from build123d import *

# Parameters (mm, degrees)
F2_R     = 32
F2_R_2   = 12
F3_DEPTH = 5
F4_R     = 5
F5_DEPTH = 5


with BuildPart() as f1:
    # F0 (on Front) → F1 (revolve)
    with BuildSketch(Plane.XZ):
        Polygon((-100, 0), (-100, 200), (-10, 275.518966806), (-10, 315.518966806), (-12, 315.518966806), (-12, 276.4515821223), (-102, 200.9326153163), (-102, -2), (0, -2), (0, 0), align=None)
    revolve(axis=Axis((0, 0, 120), (0, 0, 1)))

    # F2 (on face) → F3 (join)
    with BuildSketch(Plane.XY.offset(315.518966806)):
        Circle(F2_R)
        Circle(F2_R_2, mode=Mode.SUBTRACT)
    extrude(amount=-F3_DEPTH)

    # F4 (on face) → F5 (cut, through all)
    with BuildSketch(Plane.XY.offset(315.518966806)):
        with Locations((0, 20)):
            Circle(F4_R)
        with Locations((-20, 0)):
            Circle(F4_R)
        with Locations((0, -20)):
            Circle(F4_R)
        with Locations((20, 0)):
            Circle(F4_R)
    extrude(amount=-F5_DEPTH, mode=Mode.SUBTRACT)


solid = f1.part
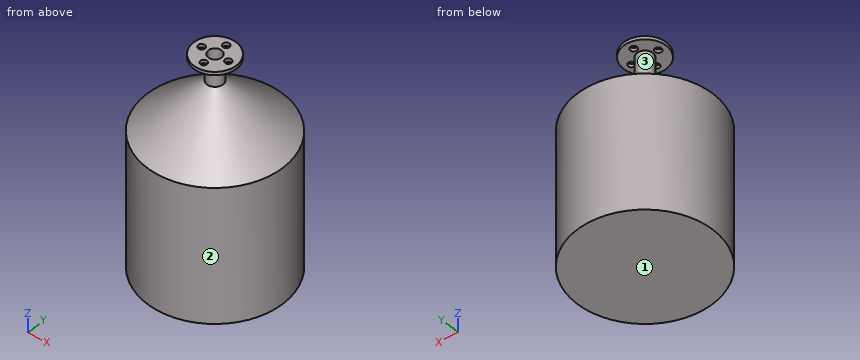
Here's how the part is built. I have some questions about the finished solid (model axes, mm). Face numbers are marked on the shaded views. Coordinates: 2 decimals unless noted, no trailing zeros. Write each loop counter-clockwise with the first axis right and the second up, starting at its lowest first coordinate (ties: lowest second). Pieces come first, ordered by that corner, then holes.
Item 1: If we mould it in two halves opening along Z, with no side actions, what happens to the marked faces 1, 2 and 3? For each: +Z half, -Z half, draft (parallel to the pull), parting line (faces both ways), or undercut.
Item 2: I want a section at C-C on z = 104.5. Write out the boundary of the cut face in (x, y), and give its area (3 significant figures).
Item 3: I want a section at A-A on x = 0. Write out the boundary of the cut face in (y, z).
Item 4: If I drill on line 1 (Y direction, x = 0, z = 312); line 2 (Y direction, x = -0.5, z = 112), over which ranges is the centre line in solid material (lowest first)?
Item 5: I want a section at D-D on z = 284.5. Write out the boundary of the cut face in (x, y).
Item 6: Will these pins go through, and if not, where does the flat tip stop? pin 1 (6 mm diameter, centred on x = 19.5, z = 85.5, fed in from +Y); pin 2 (3 mm diameter, centred on y = 26.5, z = 203.5, fed in from -X); pin 3 (2 mm diameter, centred on y = 69, z = 129.5, fed in from -X); pin 4 (8 mm diameter, centred on x = -28, z = 272.5, fed in from -Y).
Findings below:
1. face 1: -Z half
1. face 2: draft
1. face 3: undercut
2. outline: circle Ø204 at (0, 0); hole circle Ø200 at (0, 0)
2. area: 1,270 mm2
3. outline: (-102, -2) - (102, -2) - (102, 200.93) - (12, 276.45) - (12, 310.52) - (15, 310.52) - (15, 315.52) - (10, 315.52) - (10, 275.52) - (100, 200) - (100, 0) - (-100, 0) - (-100, 200) - (-10, 275.52) - (-10, 315.52) - (-15, 315.52) - (-15, 310.52) - (-12, 310.52) - (-12, 276.45) - (-102, 200.93) - close; (-32, 310.52) - (-25, 310.52) - (-25, 315.52) - (-32, 315.52) - close; (25, 310.52) - (32, 310.52) - (32, 315.52) - (25, 315.52) - close
4. line 1: y = -32 to -25, -15 to -10, 10 to 15, 25 to 32
4. line 2: y = -102 to -100, 100 to 102
5. outline: circle Ø24 at (0, 0); hole circle Ø20 at (0, 0)
6. pin 1: stops at y = 100.66
6. pin 2: stops at x = -97.22
6. pin 3: stops at x = -76.03
6. pin 4: passes through
